```python
from build123d import *

# Parameters (mm, degrees)
SKETCH1_R               = 76
SKETCH1_R_2             = 69
BOSS_EXTRUDE3_DEPTH     = 360
SKETCH2_W               = 50
SKETCH2_H               = 50
SKETCH2_W_2             = 60
CUT_EXTRUDE1_DEPTH      = 125
CUT_EXTRUDE1_DEPTH_BACK = 135
SKETCH3_W               = 60
SKETCH3_H               = 50
SKETCH3_W_2             = 50
CUT_EXTRUDE3_DEPTH      = 196
CUT_EXTRUDE3_DEPTH_BACK = 244
CUT_EXTRUDE4_DEPTH      = 404


with BuildPart() as part:
    # Sketch1 → Boss-Extrude3 (new body)
    with BuildSketch(Plane(origin=(0, 0, 0), x_dir=(0, 0, -1), z_dir=(1, 0, 0))):
        Circle(SKETCH1_R)
        Circle(SKETCH1_R_2, mode=Mode.SUBTRACT)
    extrude(amount=BOSS_EXTRUDE3_DEPTH)

    # Sketch2 → Cut-Extrude1 (cut, two sides)
    with BuildSketch(Plane(origin=(0, 0, 0), x_dir=(1, 0, 0), z_dir=(0, 1, 0))) as cut_extrude1_sk:
        with Locations((75, 51)):
            Rectangle(SKETCH2_W, SKETCH2_H)
        with Locations((285, 51)):
            Rectangle(SKETCH2_W, SKETCH2_H)
        with Locations((180, 51)):
            Rectangle(SKETCH2_W_2, SKETCH2_H)
    extrude(amount=CUT_EXTRUDE1_DEPTH, mode=Mode.SUBTRACT)
    extrude(cut_extrude1_sk.sketch, amount=-CUT_EXTRUDE1_DEPTH_BACK, mode=Mode.SUBTRACT)

    # Sketch3 → Cut-Extrude3 (cut, two sides)
    with BuildSketch(Plane(origin=(0, 0, 0), x_dir=(1, 0, 0), z_dir=(0, 1, 0))) as cut_extrude3_sk:
        with Locations((180, -51)):
            Rectangle(SKETCH3_W, SKETCH3_H)
        with Locations((75, -51)):
            Rectangle(SKETCH3_W_2, SKETCH3_H)
        with Locations((285, -51)):
            Rectangle(SKETCH3_W_2, SKETCH3_H)
    extrude(amount=CUT_EXTRUDE3_DEPTH, mode=Mode.SUBTRACT)
    extrude(cut_extrude3_sk.sketch, amount=-CUT_EXTRUDE3_DEPTH_BACK, mode=Mode.SUBTRACT)

    # Sketch4 → Cut-Extrude4 (cut)
    with BuildSketch(Plane.ZY):
        with BuildLine():
            Line((-69.189205769, -21.658804332), (-65.512565168, -21.658804332))
            ThreePointArc((-65.512565168, -21.658804332), (-66.210745314, -19.420020724), (-66.832442974, -17.158804332))
            Line((-66.832442974, -17.158804332), (-69.189205769, -17.158804332))
            Line((-69.189205769, -17.158804332), (-69.189205769, -21.658804332))
        make_face()
        with BuildLine():
            Line((-57.5, -38.141185089), (-57.5, -44.158804332))
            Line((-57.5, -44.158804332), (-53.018864567, -44.158804332))
            ThreePointArc((-53.018864567, -44.158804332), (-55.341284695, -41.210947676), (-57.5, -38.141185089))
        make_face()
        with BuildLine():
            ThreePointArc((57.5, -38.141185089), (55.341284695, -41.210947676), (53.018864567, -44.158804332))
            Line((53.018864567, -44.158804332), (57.5, -44.158804332))
            Line((57.5, -44.158804332), (57.5, -38.141185089))
        make_face()
        with BuildLine():
            ThreePointArc((66.832442974, -17.158804332), (66.210745314, -19.420020724), (65.512565168, -21.658804332))
            Line((65.512565168, -21.658804332), (69.189205769, -21.658804332))
            Line((69.189205769, -21.658804332), (69.189205769, -17.158804332))
            Line((69.189205769, -17.158804332), (66.832442974, -17.158804332))
        make_face()
    extrude(amount=-CUT_EXTRUDE4_DEPTH, mode=Mode.SUBTRACT)


solid = part.part
```
Source: CAD feature listing. Evaluate the final solid. Frame: model axes, mm. A direction names the side the tool comes from. Give positions to 0.01 mm unless a question says otherwise; leave off trailing zeros. Order: outer loops, then holes, each group sorted by start corner. A loop starts at its lowest first (then second) coordinate and runs counter-clockwise, first axis right, second up.
(1) Section query B-B (y = 0). State how many separate pieces and enclosed holes the cut face has, plus the area to 3 significant figures.
(2) Pull-direction query (Z, two-part tool) for faces 1 (the face through (180, -68, -26)), 2 (the face through (100, 16, 70)), 3 (the face through (75, 68, 26)), 4 (the face through (234.65, -30.28, -62)); classes: +Z half, -Z half, draft (parallel to the pull), parting line (faces both ways), or undercut.
(3) Contact query for flat-ended pins moving along their axis: P1, Ø4, axis at x = 245, y = -43.5, coming from the -Z side; P2, Ø3, axis at x = 195, z = 3.5, coming from the +Y side; P3, Ø5, axis at x = 101.5, z = -9, coming from the +Y side. Output: stop coordinate, or through.
(4) Material intervals for line 1 along X through (y, z) = (46.5, 56); line 2 along Z through (x, y) = (253, 62.5); line 3 along Y through (x, z) = (228.5, -28), sorted ascending.
(5) Section query C-C (x = 192). Return the cut outline in (y, z), plus the area to 3 significant figures.
(6) Access query for faces 5 (the face through (180, 68, 26)), 6 (the face through (0, -67.2, -16.5)), 7 (the face through (24.65, -30.051, 62.112)), 8 (the face through (75, 68, -26)). Directions: +Z, -Z, +X, -X, +Y, -Y. A direction counts if a zero-diameter tool reaches every point of the face in a straight line with its end or side. Return the directions, or none.
(7) Section query A-A (z = 0). Return the cut outline in (x, y), plus the area to 3 significant figures.
Outcome:
1. separate pieces: 8
1. enclosed holes: 0
1. area: 2,800 mm2
2. face 1: -Z half
2. face 2: draft
2. face 3: +Z half
2. face 4: undercut
3. P1: stops at z = -63.67
3. P2: stops at y = 75.97
3. P3: stops at y = 75.72
4. line 1: x = 0 to 50, 100 to 150, 210 to 260, 310 to 360
4. line 2: z = -43.24 to -29.24, 29.24 to 43.24
4. line 3: y = -70.65 to -63.06, 63.06 to 70.65
5. outline: (-71.41, -26) - (-63.91, -26) arc R69 cw to (-63.91, 26) - (-71.41, 26) arc R76 ccw to start; (63.91, -26) - (71.41, -26) arc R76 ccw to (71.41, 26) - (63.91, 26) arc R69 cw to start
5. area: 745 mm2
6. face 5: +Z, +Y, -Y
6. face 6: +Z, -Z, -X, +Y, -Y
6. face 7: +X, -X
6. face 8: -Z, +Y, -Y
7. outline: (0, -76) - (360, -76) - (360, -69) - (0, -69) - close; (0, 69) - (360, 69) - (360, 76) - (0, 76) - close
7. area: 5,040 mm2
